Work out the finished part from the listing and answer in its coordinate system (mm). Face numbers are marked on the shaded views. A direction names the side the tool comes from. Round coordinates to 2 decimals unless told otherwise and drop trailing zeros. Write each loop counter-clockwise with the first axis right and the second up, starting at its lowest first coordinate (ties: lowest second). Pieces come first, ordered by that corner, then holes.
from build123d import *

# Parameters (mm, degrees)
ESBO_O1_W                = 55
ESBO_O1_H                = 58
BASE_DEPTH               = 1.2
ESBO_O2_W                = 55
ESBO_O2_H                = 58
ESBO_O2_W_2              = 52
ESBO_O2_H_2              = 55
PAREDES_DEPTH            = 24
ESBO_O3_W                = 4.971937724
ESBO_O3_H                = 55
CORTE_EXTRUS_O1_DEPTH    = 24
ESBO_O4_W                = 9.2
ESBO_O4_H                = 15
ENCAIXE_CHAVE_DEPTH      = 17
ESBO_O5_W                = 1.5
ESBO_O5_H                = 18
CORTE_EXTRUS_O3_DEPTH    = 68.089790579
FILETE1_R                = 8
FILETE2_R                = 3
CHANFRO1_SIZE            = 1
CORTE_EXTRUS_O5_DEPTH    = 17
ESBO_O8_W                = 55
ESBO_O8_H                = 18
CORTE_EXTRUS_O6_DEPTH    = 17
FILETE6_R                = 8
FILETE7_R                = 10
ESBO_O9_W                = 12
ESBO_O9_H                = 1.2
RESSALTO_EXTRUS_O3_DEPTH = 10
ESBO_O10_R               = 1.6
CORTE_EXTRUS_O7_DEPTH    = 10
FILETE8_R                = 3
FILETE9_R                = 3
FILETE10_R               = 3
CHANFRO2_SIZE            = 0.5


with BuildPart() as part:
    # Esboço1 → Base (new body)
    with BuildSketch(Plane(origin=(0, 0, 0), x_dir=(1, 0, 0), z_dir=(0, 1, 0))):
        Rectangle(ESBO_O1_W, ESBO_O1_H)
    extrude(amount=BASE_DEPTH)

    # Esboço2 → Paredes (add)
    with BuildSketch(Plane(origin=(0, 1.2, 0), x_dir=(1, 0, 0), z_dir=(0, 1, 0))):
        Rectangle(ESBO_O2_W, ESBO_O2_H)
        Rectangle(ESBO_O2_W_2, ESBO_O2_H_2, mode=Mode.SUBTRACT)
    extrude(amount=PAREDES_DEPTH)

    # Esboço3 → Corte-extrusão1 (cut)
    with BuildSketch(Plane(origin=(0, 25.2, 0), x_dir=(1, 0, 0), z_dir=(0, 1, 0))):
        with Locations((-27.5, 0)):
            Rectangle(ESBO_O3_W, ESBO_O3_H)
    extrude(amount=-CORTE_EXTRUS_O1_DEPTH, mode=Mode.SUBTRACT)

    # Esboço4 → Encaixe chave (cut)
    with BuildSketch(Plane(origin=(0, 0, -29), x_dir=(-1, 0, 0), z_dir=(0, 0, -1))):
        with Locations((6.5, 15.2)):
            Rectangle(ESBO_O4_W, ESBO_O4_H)
    extrude(amount=-ENCAIXE_CHAVE_DEPTH, mode=Mode.SUBTRACT)

    # Esboço5 → Corte-extrusão3 (cut, through all)
    with BuildSketch(Plane.ZY.offset(27.5)):
        with Locations((28.25, 16.2)):
            Rectangle(ESBO_O5_W, ESBO_O5_H)
    extrude(amount=-CORTE_EXTRUS_O3_DEPTH, mode=Mode.SUBTRACT)

    # Filete1
    filete1_edges = [part.edges().sort_by_distance(p)[0] for p in [
        (-27.5, 25.2, -28.25),
    ]]
    fillet(filete1_edges, radius=FILETE1_R)

    # Filete2
    filete2_edges = [part.edges().sort_by_distance(p)[0] for p in [
        (-27.5, 7.2, 28.25),
    ]]
    fillet(filete2_edges, radius=FILETE2_R)

    # Chanfro1
    chanfro1_edges = [part.edges().sort_by_distance(p)[0] for p in [
        (26, 1.2, 0),
        (-0.75, 1.2, -27.5),
        (-0.75, 1.2, 27.5),
    ]]
    chamfer(chanfro1_edges, length=CHANFRO1_SIZE)

    # Esboço7 → Corte-extrusão5 (cut)
    with BuildSketch(Plane(origin=(0, 1.2, 0), x_dir=(1, 0, 0), z_dir=(0, 1, 0))):
        with BuildLine():
            Line((-14.5, -17.5), (14.5, -17.5))
            ThreePointArc((14.5, -17.5), (16.621320344, -16.621320344), (17.5, -14.5))
            Line((17.5, -14.5), (17.5, 14.5))
            ThreePointArc((17.5, 14.5), (16.621320344, 16.621320344), (14.5, 17.5))
            Line((14.5, 17.5), (-14.5, 17.5))
            ThreePointArc((-14.5, 17.5), (-16.621320344, 16.621320344), (-17.5, 14.5))
            Line((-17.5, 14.5), (-17.5, -14.5))
            ThreePointArc((-17.5, -14.5), (-16.621320344, -16.621320344), (-14.5, -17.5))
        make_face()
    extrude(amount=-CORTE_EXTRUS_O5_DEPTH, mode=Mode.SUBTRACT)

    # Esboço8 → Corte-extrusão6 (cut)
    with BuildSketch(Plane(origin=(27.5, 0, 0), x_dir=(0, 0, -1), z_dir=(1, 0, 0))):
        with Locations((0, 16.2)):
            Rectangle(ESBO_O8_W, ESBO_O8_H)
    extrude(amount=-CORTE_EXTRUS_O6_DEPTH, mode=Mode.SUBTRACT)

    # Filete6
    filete6_edges = [part.edges().sort_by_distance(p)[0] for p in [
        (27.5, 25.2, -28.25),
    ]]
    fillet(filete6_edges, radius=FILETE6_R)

    # Filete7
    filete7_edges = [part.edges().sort_by_distance(p)[0] for p in [
        (26.75, 7.2, -27.5),
    ]]
    fillet(filete7_edges, radius=FILETE7_R)

    # Esboço9 → Ressalto-extrusão3 (add)
    with BuildSketch(Plane.XY.offset(29)):
        with Locations((21.5, 0.6)):
            Rectangle(ESBO_O9_W, ESBO_O9_H)
    extrude(amount=RESSALTO_EXTRUS_O3_DEPTH)

    # Esboço10 → Corte-extrusão7 (cut)
    with BuildSketch(Plane(origin=(0, 1.2, 0), x_dir=(1, 0, 0), z_dir=(0, 1, 0))):
        with Locations(Location((21.5, -34, 0), (0, 0, 180))):
            Circle(ESBO_O10_R)
    extrude(amount=-CORTE_EXTRUS_O7_DEPTH, mode=Mode.SUBTRACT)

    # Filete8
    filete8_edges = [part.edges().sort_by_distance(p)[0] for p in [
        (15.5, 0.6, 39),
    ]]
    fillet(filete8_edges, radius=FILETE8_R)

    # Filete9
    filete9_edges = [part.edges().sort_by_distance(p)[0] for p in [
        (27.5, 0.6, 39),
    ]]
    fillet(filete9_edges, radius=FILETE9_R)

    # Filete10
    filete10_edges = [part.edges().sort_by_distance(p)[0] for p in [
        (15.5, 0.6, 29),
    ]]
    fillet(filete10_edges, radius=FILETE10_R)

    # Chanfro2
    chanfro2_edges = [part.edges().sort_by_distance(p)[0] for p in [
        (20, 1.2, 29),
    ]]
    chamfer(chanfro2_edges, length=CHANFRO2_SIZE)


solid = part.part
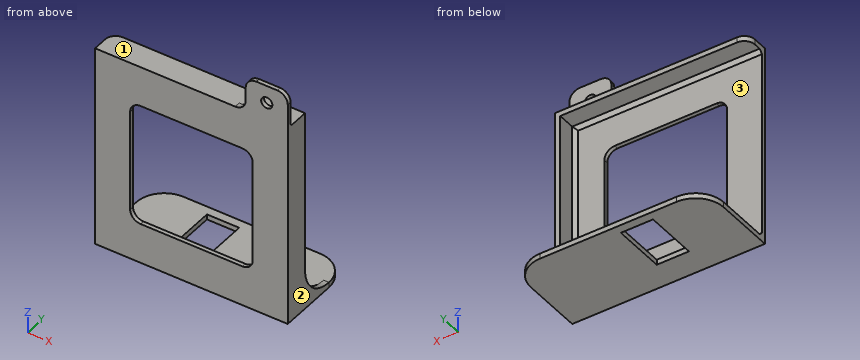
Q1. Given pin 1 (5 mm diameter, centred on x = 21.5, z = 34, fed in from +Y); pin 2 (12 mm diameter, centred on y = 12, z = 9.5, fed in from -X); pin 3 (0.8 mm diameter, centred on y = 19, z = -28, fed in from +X); pin 4 (4 mm diameter, centred on x = -22, z = 32, fed in from +Y), each flat-ended and moving along its own axis, determine where each tip first touches the part or whether it passes through.
Q2. Find the intervals of material crossed by L1, parallel to Z at x = 21.5, y = 0.4; L2, parallel to Z at x = 6.5, y = 6.25; L3, parallel to Y at x = -24, z = 23.5, in increasing order.
Q3. Find section B-B (x = -1). Determine the outline of the cut face in (y, z), plus the area to 3 significant figures.
Q4. Find section C-C (z = 19). Determine the outline of the cut face in (x, y).
Q5. Find section D-D (y = 21.5). Determine the outline of the cut face in (x, z).
Q6. A tool of negligible diameter and unlimited length cuts with its end or side. For the marked faces 1, 2 and 3, from which of +Z, -Z, +X, -X, +Y, -Y can it reach the whole face along a straight path? Write none if from no direction.
Q7. Find section A-A (z = 34). Determine the outline of the cut face in (x, y).
Report:
1. pin 1: stops at y = 1.2
1. pin 2: stops at x = 26
1. pin 3: stops at x = 27.38
1. pin 4: passes through
2. L1: z = -29 to 32.4, 35.6 to 39
2. L2: z = -29 to -27.5, 27.5 to 29
2. L3: y = 0 to 1.2
3. outline: (0, -29) - (25.2, -29) - (25.2, -27.5) - (2.2, -27.5) - (1.2, -26.5) - (1.2, -17.5) - (0, -17.5) - close; (0, 17.5) - (1.2, 17.5) - (1.2, 26.5) - (2.2, 27.5) - (7.2, 27.5) - (7.2, 29) - (0, 29) - close
3. area: 73.6 mm2
4. outline: (-27.5, 0) - (27.5, 0) - (27.5, 7.2) - (26, 7.2) - (26, 2.2) - (25, 1.2) - (-27.5, 1.2) - close
5. outline: (-26.25, -29) - (-11.1, -29) - (-11.1, -27.5) - (-26.25, -27.5) - close; (-1.9, -29) - (26.25, -29) - (26.25, -27.5) - (-1.9, -27.5) - close
6. face 1: +Z, -X, +Y
6. face 2: +Z, -Z, +X, +Y, -Y
6. face 3: -X, +Y
7. outline: (15.5, 0) - (19.9, 0) - (19.9, 1.2) - (15.5, 1.2) - close; (23.1, 0) - (27.5, 0) - (27.5, 1.2) - (23.1, 1.2) - close
